Read the model definition and answer for the solid it produces. Units are mm, in the model's axes. A direction names the side the tool comes from. Coordinates: 2 decimals unless noted, no trailing zeros. Order: outer loops, then holes, each group sorted by start corner. A loop starts at its lowest first (then second) coordinate and runs counter-clockwise, first axis right, second up. Notation, with made-up numbers: M 54.5,61.5 L 65.5,61.5 A23 ccw 65.5,81.5 Z; hole C 53,77 d11. An arc over 180 degrees is marked long. Write each question's results on one line, items separated by ' | '.
```python
from build123d import *

# Parameters (mm, degrees)
SKETCH_1_R          = 25
EXTRUDE_1_DEPTH     = 15
SKETCH_2_R          = 15.2
CUT_EXTRUDE_1_DEPTH = 8
SKETCH_3_R          = 2.15
CUT_EXTRUDE_2_DEPTH = 10
CUT_EXTRUDE_3_DEPTH = 39.405728739


with BuildPart() as part:
    # 草图1 → 凸台-拉伸1 (new body)
    with BuildSketch(Plane.XY):
        Circle(SKETCH_1_R)
    extrude(amount=EXTRUDE_1_DEPTH)

    # 草图2 → 切除-拉伸1 (cut)
    with BuildSketch(Plane(origin=(0, 0, 0), x_dir=(-1, 0, 0), z_dir=(0, 0, -1))):
        Circle(SKETCH_2_R)
    extrude(amount=-CUT_EXTRUDE_1_DEPTH, mode=Mode.SUBTRACT)

    # 草图3 → 切除-拉伸2 (cut)
    with BuildSketch(Plane.XY.offset(15)):
        with Locations((-14.278039738, -7.313917654)):
            Circle(SKETCH_3_R)
        with Locations((-7.586084988, 14.301302484)):
            Circle(SKETCH_3_R)
        with Locations((14.029135151, 7.609347734)):
            Circle(SKETCH_3_R)
        with Locations((7.3371804, -14.005872405)):
            Circle(SKETCH_3_R)
    extrude(amount=-CUT_EXTRUDE_2_DEPTH, mode=Mode.SUBTRACT)

    # 草图4 → 切除-拉伸3 (cut, through all)
    with BuildSketch(Plane.XY.offset(15)):
        with BuildLine():
            ThreePointArc((3.925547706, 0.14771504), (2.811003713, 2.937983491), (0.080807938, 4.192510243))
            Line((0.080807938, 4.192510243), (-4.105054455, 0.894244634))
            ThreePointArc((-4.105054455, 0.894244634), (-0.499326438, -3.88489818), (3.925547706, 0.14771504))
        make_face()
    extrude(amount=-CUT_EXTRUDE_3_DEPTH, mode=Mode.SUBTRACT)


solid = part.part
```
(1) For faces 1 (the cylindrical face through (15.185, 0.668, 3.944)), 2 (the flat face through (11, -11, 0)), 3 (the flat face through (-1.98, 2.57, 11.55)), 4 (the cylindrical face through (-16.426, -7.219, 10.07)), determine the directions among +Z, -Z, +X, -X, +Y, -Y from which every point of the face is accessible in a straight line to the end or side of a thin tool.
Conclusion:
face 1: -Z | face 2: -Z, +X, -X, +Y, -Y | face 3: +Z, -Z | face 4: +Z
(2) The part is cut by section B-B, the plane z = 10.25. Write down the section's boundary in (x, y), then the cut area to 3 significant figures.
Conclusion:
outline: C 0,0 d50; hole C -14.28,-7.31 d4.3; hole C -7.59,14.3 d4.3; hole M -4.11,0.89 A4.05 ccw long 0.08,4.19 Z; hole C 7.34,-14.01 d4.3; hole C 14.03,7.61 d4.3 | area: 1,860 mm²
(3) Given pin 1 (1.9 mm diameter, centred on x = 6.5, y = -13.5, fed in from +Z); pin 2 (15 mm diameter, centred on x = -0.5, y = -6.5, fed in from -Z); pin 3 (2 mm diameter, centred on x = 11.5, z = 7.5, fed in from +Y), each flat-ended and moving along its own axis, determine where each tip first touches the part or whether it passes through.
Conclusion:
pin 1: z = 5 | pin 2: z = 8 | pin 3: y = 22.69
(4) The part is cut by section A-A, the plane x = 2.5. Write down the section's boundary in (y, z), then the cut area to 3 significant figures.
Conclusion:
outline: M -24.87,0 L -14.99,0 L -14.99,8 L -2.94,8 L -2.94,15 L -24.87,15 Z; M 3.23,8 L 14.99,8 L 14.99,0 L 24.87,0 L 24.87,15 L 3.23,15 Z | area: 463 mm²
(5) Straight lines are drawn through the part: line 1 (Y direction, x = -0.5, z = 7.75) (3 decimals); line 2 (Z direction, x = 1, y = -14). For each, find the intervals that lie inside material, in ascending order.
Conclusion:
line 1: -24.995 to -15.192, 15.192 to 24.995 | line 2: 8 to 15
(6) The mould has two halves that part along X. Classify faces 5 (the cylindrical face through (23.846, 7.509, 7.395)), 6 (the flat face through (8, -15, 5)), 7 (the flat face through (0, -5, 15)): pulls with the +X half, pulls with the -X half, needs draft (parallel to the pull), parting line crosses it, or undercut.
Conclusion:
face 5: parting line crosses it | face 6: undercut | face 7: needs draft
(7) The part is cut by section C-C, the plane y = 3. Write down the section's boundary in (x, z), then the cut area to 3 significant figures.
Conclusion:
outline: M -24.82,0 L -14.9,0 L -14.9,8 L -1.43,8 L -1.43,15 L -24.82,15 Z; M 2.75,8 L 14.9,8 L 14.9,0 L 24.82,0 L 24.82,15 L 2.75,15 Z | area: 477 mm²
(8) The part is cut by section D-D, the plane z = 1.25. Write down the section's boundary in (x, y), then the cut area to 3 significant figures.
Conclusion:
outline: C 0,0 d50; hole C 0,0 d30.4 | area: 1,240 mm²
